Check sheet for the modelled part. Datum: model origin and axes. Units: mm. A direction names the side the tool comes from. Give positions to 0.01 mm unless a question says otherwise; leave off trailing zeros. Order: outer loops, then holes, each group sorted by start corner. A loop starts at its lowest first (then second) coordinate and runs counter-clockwise, first axis right, second up. Notation, with made-up numbers: M 11,-29.75 L 45,-29.75 A21 cw 45,-11.75 Z; hole C 53,14.25 d3. An arc over 180 degrees is marked long. Return JSON: item names as keys, results as strings. Group by question number.
Autodesk Inventor part; units mm, degrees
ref_plane "YZ Plane" through (0, 0, 0) normal (1, 0, 0) x (0, 1, 0)
ref_plane "XZ Plane" through (0, 0, 0) normal (0, 1, 0) x (-1, 0, 0)
ref_plane "XY Plane" through (0, 0, 0) normal (0, 0, 1) x (1, 0, 0)
sketch "Sketch1" plane through (0, 0, 0) normal (0, 0, 1) x (1, 0, 0)
  line L0 (0, 0) -> (0, 15.875)
  line L1 (0, 15.875) -> (0.7937, 15.875)
  line L2 (0.7937, 15.875) -> (0.7938, 0.7937)
  line L3 (0.7938, 0.7937) -> (15.875, 0.7937)
  line L4 (15.875, 0.7937) -> (15.875, 0)
  line L5 (15.875, 0) -> (0, 0)
  dimension "d0" = 15.875
  dimension "d1" = 0.7937
extrude "Extrusion1" add sketch "Sketch1" along normal blind 481.8063
sketch "Sketch2" plane through (0, 0, 0) normal (-1, 0, 0) x (0, 0, 1)
  circle A0 centre (46.4113, 9.6145) radius 3.3782
  circle A1 centre (158.9314, 9.6145) radius 3.3782
  circle A2 centre (701.675, 21.658) radius 3.3782 construction
  circle A3 centre (701.675, 43.7923) radius 3.3782 construction
  circle A4 centre (701.675, 32.7252) radius 3.3782 construction
  circle A5 centre (701.675, 10.5909) radius 3.3782
  line L0 (366.395, 51.5938) -> (366.395, 0.7938) construction
  line L1 (708.025, 0.7938) -> (366.395, 0.7938) construction
  line L2 (708.025, 51.5938) -> (708.025, 0.7938) construction
  line L3 (366.395, 51.5938) -> (708.025, 51.5938) construction
  circle A6 centre (219.075, 21.658) radius 3.3782 construction
  circle A7 centre (219.075, 43.7923) radius 3.3782 construction
  circle A8 centre (219.075, 32.7252) radius 3.3782 construction
  circle A9 centre (219.075, 10.5909) radius 3.3782
  line L4 (262.255, 51.5938) -> (262.255, 0.7938) construction
  line L5 (212.725, 0.7938) -> (262.255, 0.7938) construction
  line L6 (212.725, 0.7938) -> (212.725, 51.5938) construction
  line L7 (212.725, 51.5938) -> (262.255, 51.5938) construction
  line L8 (0, 0) -> (0, 15.875)
  line L9 (481.8063, 15.875) -> (481.8063, 0)
  line L10 (19.05, -173.8312) -> (19.05, -103.9812) construction
  line L11 (19.05, -103.9812) -> (285.75, -103.9812) construction
  line L12 (285.75, -103.9812) -> (285.75, -173.8312) construction
  line L13 (285.75, -173.8312) -> (19.05, -173.8312) construction
  line L14 (38.1, -294.4812) -> (38.1, -265.9062) construction
  line L15 (38.1, -265.9062) -> (285.75, -265.9062) construction
  line L16 (285.75, -265.9062) -> (285.75, -294.4812) construction
  line L17 (285.75, -294.4812) -> (38.1, -294.4812) construction
  circle A10 centre (593.725, 76.9938) radius 3.3782 construction
  circle A11 centre (314.325, -202.4062) radius 3.3782 construction
  circle A12 centre (454.025, 76.9938) radius 3.3782 construction
  circle A13 centre (417.4958, -17.1968) radius 3.3782 construction
  circle A14 centre (408.5156, -26.1771) radius 3.3782 construction
  circle A15 centre (516.3297, -116.0307) radius 3.3782 construction
  circle A16 centre (507.3495, -125.011) radius 3.3782 construction
  circle A17 centre (259.0504, -62.7062) radius 3.3782 construction
  circle A18 centre (314.325, -62.7062) radius 3.3782 construction
  line L18 (191.2043, 15.9645) -> (11.4863, 15.9645) construction
  line L19 (11.4863, 15.9645) -> (11.4863, 0.7938) construction
  line L20 (11.4863, 0.7938) -> (0, 0.7938) construction
  line L21 (0, 0.7938) -> (0, -316.7062) construction
  line L22 (0, -316.7062) -> (307.975, -316.7062) construction
  line L23 (307.975, -316.7062) -> (307.975, -208.7562) construction
  line L24 (307.975, -208.7562) -> (314.325, -208.7562) construction
  arc A19 (314.325, -208.7562) -> (600.075, 76.9938) centre (314.325, 76.9938) ccw construction
  line L25 (600.075, 76.9938) -> (600.075, 83.3438) construction
  line L26 (600.075, 83.3438) -> (587.375, 83.3438) construction
  line L27 (587.375, 83.3438) -> (587.375, 76.9938) construction
  arc A20 (314.325, -196.0562) -> (587.375, 76.9938) centre (314.325, 76.9938) ccw construction
  line L28 (314.325, -196.0562) -> (314.325, -69.0562) construction
  arc A21 (314.325, -69.0562) -> (460.375, 76.9938) centre (314.325, 76.9938) ccw construction
  line L29 (460.375, 76.9938) -> (460.375, 83.3438) construction
  line L30 (460.375, 83.3438) -> (447.675, 83.3438) construction
  line L31 (447.675, 83.3438) -> (447.675, 76.9938) construction
  arc A22 (314.325, -56.3562) -> (447.675, 76.9938) centre (314.325, 76.9938) ccw construction
  line L32 (314.325, -56.3562) -> (193.675, 0.7938) construction
  line L33 (193.675, 0.7938) -> (193.675, 13.4938) construction
  line L34 (193.675, 13.4938) -> (191.2043, 15.9645) construction
  line L35 (19.05, -215.1062) -> (19.05, -186.5312) construction
  line L36 (19.05, -186.5312) -> (285.75, -186.5312) construction
  line L37 (285.75, -186.5312) -> (285.75, -215.1062) construction
  line L38 (285.75, -215.1062) -> (19.05, -215.1062) construction
  line L39 (25.4, -253.2062) -> (25.4, -281.7812) construction
  line L40 (25.4, -281.7812) -> (19.05, -281.7812) construction
  line L41 (19.05, -281.7812) -> (19.05, -253.2062) construction
  line L42 (19.05, -253.2062) -> (12.7, -253.2062) construction
  line L43 (12.7, -253.2062) -> (12.7, -227.8062) construction
  line L44 (12.7, -227.8062) -> (215.9, -227.8062) construction
  line L45 (215.9, -227.8062) -> (215.9, -253.2062) construction
  line L46 (215.9, -253.2062) -> (25.4, -253.2062) construction
  line L47 (25.4, 6.4395) -> (25.4, -62.7062) construction
  line L48 (25.4, -62.7062) -> (215.9, -62.7062) construction
  line L49 (215.9, -62.7062) -> (215.9, -88.1062) construction
  line L50 (215.9, -88.1062) -> (12.7, -88.1062) construction
  line L51 (12.7, -88.1062) -> (12.7, -62.7062) construction
  line L52 (12.7, -62.7062) -> (19.05, -62.7062) construction
  line L53 (19.05, -62.7062) -> (19.05, 6.4395) construction
  line L54 (19.05, 6.4395) -> (25.4, 6.4395) construction
  circle A23 centre (238.125, -310.3562) radius 3.3782 construction
  circle A24 centre (219.075, -310.3562) radius 3.3782 construction
  circle A25 centre (46.4113, 9.6145) radius 3.3782 construction
  circle A26 centre (158.9314, 9.6145) radius 3.3782 construction
  arc A27 (314.325, -62.7062) -> (454.025, 76.9938) centre (314.325, 76.9938) ccw construction
  line L55 (481.8063, 7.9375) -> (0, 7.9375) construction
  circle A28 centre (435.7636, 7.9375) radius 3.3782
  dimension "d6" = 6.7564
extrude "Extrusion2" cut sketch "Sketch2" against normal through all
properties part number "Shooter Middle Support Bar" material "Aluminum 6061"
1) Sectioned sample at B-B on x = 7.5. Record the boundary of the cut face in (y, z).
2) Sectioned sample at A-A on z = 334.5. Record the boundary of the cut face in (x, y) (3 decimals), then the cut area to 3 significant figures.
3) Depth check by flat-ended pin: P1, Ø6, axis at y = 7.94, z = 435.76, coming from the +X side; P2, Ø1.5, axis at y = 13, z = 98, coming from the +X side; P3, Ø3, axis at x = 2.5, z = 192, coming from the +Y side; P4, Ø9, axis at y = 10.59, z = 219.08, coming from the -X side. Enter the tip coordinate at first touch or a pass-through.
4) Tool access check on faces 1 (the face through (8, 0.794, 238)), 2 (the face through (4.4, 0.3, 0)). Record the directions out of +Z, -Z, +X, -X, +Y, -Y that give a thin tool (end or side, any length) a straight path to the whole face; none if there is none.
5) Material ranges on line 1 along Y through (x, z) = (9.75, 394), recorded low to high.
Reply:
{
 "1": {"outline": "M 0,0 L 0.79,0 L 0.79,481.81 L 0,481.81 Z"},
 "2": {"outline": "M 0,0 L 15.875,0 L 15.875,0.794 L 0.794,0.794 L 0.794,15.875 L 0,15.875 Z", "area": "24.6 mm^2"},
 "3": {"P1": "through", "P2": "x = 0.79", "P3": "y = 0.79", "P4": "x = 0"},
 "4": {"face 1": "+Z, -Z, +X, +Y", "face 2": "-Z, +X, -X, +Y, -Y"},
 "5": {"line 1": "0 to 0.79"}
}
